Read the model definition and answer for the solid it produces. Units are mm, in the model's axes. Face numbers are marked on the shaded views. A direction names the side the tool comes from. Coordinates: 2 decimals unless noted, no trailing zeros. Order: outer loops, then holes, each group sorted by start corner. A loop starts at its lowest first (then second) coordinate and runs counter-clockwise, first axis right, second up. Notation, with made-up numbers: M 70,50.5 L 89,50.5 A20 ccw 89,82.5 Z; hole C -8.5,5 d9. An arc over 180 degrees is marked long. One line per question, with ' | ' between items. Start each with the question number.
1) The mould has two halves that part along Y. Classify the marked faces 1, 2, 3 and 4: +Y half, -Y half, draft (parallel to the pull), parting line (faces both ways), or undercut.
2) Find section D-D, the plane y = 30.5. Write down the section's boundary in (x, z) (3 decimals).
3) Find section B-B, the plane z = 6.5. Write down the section's boundary in (x, y), plus the area to 3 significant figures.
4) Find section C-C, the plane x = 0. Write down the section's boundary in (y, z), plus the area to 3 significant figures.
5) A tool of negligible diameter and unlimited length cuts with its end or side. For the marked faces 5 and 6, from which of +Z, -Z, +X, -X, +Y, -Y can it reach the whole face along a straight path? Write none if from no direction.
6) Given P1, Ø0.9, axis at x = -10.5, z = 2, coming from the -Y side; P2, Ø2, axis at x = -11.5, y = 34.5, coming from the -Z side, each flat-ended and moving along its own axis, determine where each tip first touches the part or whether it passes through.
7) Consider probe 1 along X at (y, z) = (31.5, 7.5); probe 2 along X at (y, z) = (30, 6.5); probe 3 along X at (y, z) = (32, 1.25). Determine where each line is inside the solid, lowest interval first.
8) Find section A-A, the plane y = 34. Write down the section's boundary in (x, z).
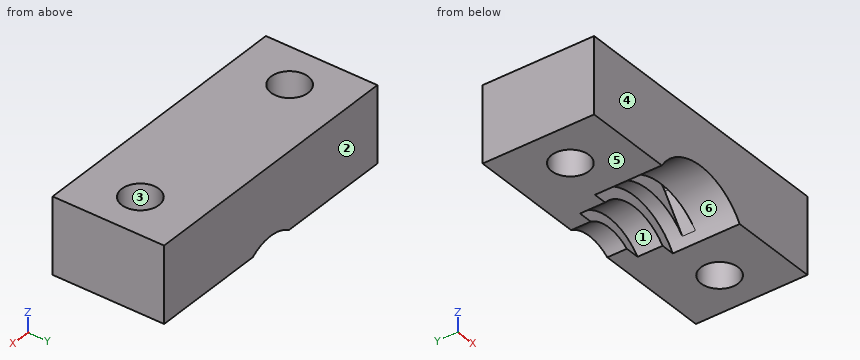
from build123d import *

# Parameters (mm, degrees)
SKETCH1_W           = 30
SKETCH1_H           = 12
SKETCH1_R           = 2
BOSS_EXTRUDE1_DEPTH = 8.2
SKETCH2_R           = 6.5
CUT_EXTRUDE1_DEPTH  = 7.2
SKETCH3_R           = 5.35
CUT_EXTRUDE2_DEPTH  = 9.9
SKETCH4_R           = 4.325
CUT_EXTRUDE3_DEPTH  = 13.9
CUT_EXTRUDE4_START  = -5.7
CUT_EXTRUDE4_DEPTH  = 1.4


with BuildPart() as part:
    # Sketch1 → Boss-Extrude1 (new body)
    with BuildSketch(Plane.XY):
        with Locations((-11.682314935, 31.556218858)):
            Rectangle(SKETCH1_W, SKETCH1_H)
        with Locations((-22.182314935, 31.556218858)):
            Circle(SKETCH1_R, mode=Mode.SUBTRACT)
        with Locations((-1.182314935, 31.556218858)):
            Circle(SKETCH1_R, mode=Mode.SUBTRACT)
    extrude(amount=BOSS_EXTRUDE1_DEPTH)

    # Sketch2 → Cut-Extrude1 (cut)
    with BuildSketch(Plane(origin=(0, 25.556218858, 0), x_dir=(-1, 0, 0), z_dir=(0, -1, 0))):
        with Locations((11.682314935, 3.5)):
            Circle(SKETCH2_R)
    extrude(amount=-CUT_EXTRUDE1_DEPTH, mode=Mode.SUBTRACT)

    # Sketch3 → Cut-Extrude2 (cut)
    with BuildSketch(Plane(origin=(0, 25.556218858, 0), x_dir=(-1, 0, 0), z_dir=(0, -1, 0))):
        with Locations((11.682314935, 3.5)):
            Circle(SKETCH3_R)
    extrude(amount=-CUT_EXTRUDE2_DEPTH, mode=Mode.SUBTRACT)

    # Sketch4 → Cut-Extrude3 (cut)
    with BuildSketch(Plane(origin=(0, 25.556218858, 0), x_dir=(-1, 0, 0), z_dir=(0, -1, 0))):
        with Locations((11.682314935, 3.5)):
            Circle(SKETCH4_R)
    extrude(amount=-CUT_EXTRUDE3_DEPTH, mode=Mode.SUBTRACT)

    # Sketch5 → Cut-Extrude4 (cut)
    with BuildSketch(Plane(origin=(0, 25.556218858, 0), x_dir=(-1, 0, 0), z_dir=(0, -1, 0)).offset(CUT_EXTRUDE4_START)):
        with BuildLine():
            Line((9.270124371, -4.128630198), (5.336263245, 1.191543622))
            Line((5.336263245, 1.191543622), (18.008683121, 1.191543622))
            Line((18.008683121, 1.191543622), (14.098774847, -4.122841808))
            ThreePointArc((14.098774847, -4.122841808), (11.685911211, -5.344997844), (9.270124371, -4.128630198))
        make_face()
    extrude(amount=CUT_EXTRUDE4_DEPTH, mode=Mode.SUBTRACT)


solid = part.part
Report:
1) face 1: draft | face 2: +Y half | face 3: undercut | face 4: -Y half
2) outline: M -26.682,0 L -23.881,0 L -23.881,8.2 L -26.682,8.2 Z; M -20.484,0 L -17.16,0 A6.5 cw -16.483,0.882 L -14.099,4.123 A3 cw -9.27,4.129 L -6.814,0.807 A6.5 cw -6.205,0 L -2.881,0 L -2.881,8.2 L -20.484,8.2 Z; M 0.516,0 L 3.318,0 L 3.318,8.2 L 0.516,8.2 Z
3) outline: M -26.68,25.56 L 3.32,25.56 L 3.32,37.56 L -26.68,37.56 Z; hole C -22.18,31.56 d4; hole C -1.18,31.56 d4 | area: 335 mm^2
4) outline: M 25.56,0 L 29.94,0 L 29.94,8.2 L 25.56,8.2 Z; M 33.17,0 L 37.56,0 L 37.56,8.2 L 33.17,8.2 Z | area: 71.9 mm^2
5) face 5: -Z, +X, -X, +Y, -Y | face 6: -Z, -Y
6) P1: stops at y = 32.76 | P2: stops at z = 0.8
7) probe 1: x = -26.68 to -24.18, -20.18 to -3.18, 0.82 to 3.32 | probe 2: x = -26.68 to -23.44, -20.93 to -2.44, 0.07 to 3.32 | probe 3: x = -26.68 to -24.13, -20.23 to -16.12, -7.25 to -3.13, 0.77 to 3.32
8) outline: M -26.68,0 L -15.73,0 A5.35 cw -7.64,0 L 3.32,0 L 3.32,8.2 L -26.68,8.2 Z
